```python
from build123d import *

# Parameters (mm, degrees)
BOSS_EXTRUDE1_DEPTH = 50.8
SKETCH3_R           = 3.302
CUT_EXTRUDE1_DEPTH  = 50.8
SKETCH4_R           = 3.302
CUT_EXTRUDE2_DEPTH  = 70.633186233


with BuildPart() as part:
    # Sketch2 → Boss-Extrude1 (new body)
    with BuildSketch(Plane(origin=(0, 0, 0), x_dir=(1, 0, 0), z_dir=(0, 1, 0))):
        Polygon((0, 0), (0, -28.575), (38.1, -28.575), (38.1, 0), (34.925, 0), (34.925, -25.4), (3.175, -25.4), (3.175, 0), align=None)
    extrude(amount=BOSS_EXTRUDE1_DEPTH)

    # Sketch3 → Cut-Extrude1 (cut)
    with BuildSketch(Plane(origin=(0, 0, 25.4), x_dir=(-1, 0, 0), z_dir=(0, 0, -1))):
        with Locations((-19.685, 12.7)):
            Circle(SKETCH3_R)
        with Locations((-19.685, 38.091107032)):
            Circle(SKETCH3_R)
    extrude(amount=-CUT_EXTRUDE1_DEPTH, mode=Mode.SUBTRACT)

    # Sketch4 → Cut-Extrude2 (cut, through all)
    with BuildSketch(Plane(origin=(38.1, 0, 0), x_dir=(0, 0, -1), z_dir=(1, 0, 0))):
        with Locations((-11.90625, 38.1)):
            Circle(SKETCH4_R)
        with Locations((-11.90625, 12.7)):
            Circle(SKETCH4_R)
    extrude(amount=-CUT_EXTRUDE2_DEPTH, mode=Mode.SUBTRACT)


solid = part.part
```
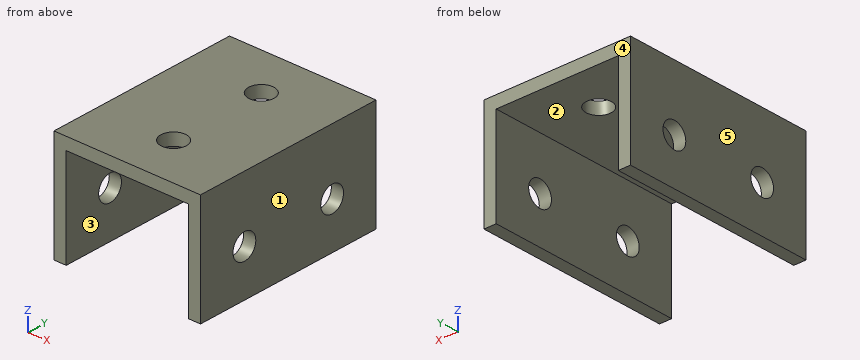
Can you work these out from the model? Positions are in its coordinate system, mm. Face numbers are marked on the shaded views. A direction names the side the tool comes from. Coordinates: 2 decimals unless noted, no trailing zeros. Order: outer loops, then holes, each group sorted by start corner. A loop starts at its lowest first (then second) coordinate and runs counter-clockwise, first axis right, second up. Notation, with made-up numbers: (36, -14.5) -> (42, -14.5) arc R22 ccw to (42, 1.5) -> close; hole circle Ø2 at (-33, 82). An arc over 180 degrees is marked (long way). Write each question's results on one line, items separated by ' | '.
Item 1: I want a section at B-B, the plane y = 12.7. Write out the boundary of the cut face in (x, z) (3 decimals), then the cut area to 3 significant figures.
Results are:
outline: (0, 0) -> (3.175, 0) -> (3.175, 8.604) -> (0, 8.604) -> close; (0, 15.208) -> (3.175, 15.208) -> (3.175, 25.4) -> (16.383, 25.4) -> (16.383, 28.575) -> (0, 28.575) -> close; (22.987, 25.4) -> (34.925, 25.4) -> (34.925, 15.208) -> (38.1, 15.208) -> (38.1, 28.575) -> (22.987, 28.575) -> close; (34.925, 0) -> (38.1, 0) -> (38.1, 8.604) -> (34.925, 8.604) -> close | area: 219 mm²
Item 2: If I drill on line 1 along X through (y, z) = (31, 21.5) (3 decimals); line 2 along Z through (x, y) = (24.5, 49) (3 decimals), over which ranges is the centre line in solid material (lowest first)?
Results are:
line 1: 0 to 3.175, 34.925 to 38.1 | line 2: 25.4 to 28.575
Item 3: I want a section at D-D, the plane y = 24. Write out the boundary of the cut face in (x, z) (3 decimals).
Results are:
outline: (0, 0) -> (3.175, 0) -> (3.175, 25.4) -> (34.925, 25.4) -> (34.925, 0) -> (38.1, 0) -> (38.1, 28.575) -> (0, 28.575) -> close
Item 4: I'm going to push flat-ended pins straight in: pin 1 Ø8.5 at (x, y) = (19.685, 12.7) entering from +Z (3 decimals); pin 2 Ø4 at (y, z) = (12.7, 11.91) entering from +X; pin 3 Ø12 at (x, y) = (25.5, 19) entering from -Z. Where does each tip first touch, or does it pass through?
Results are:
pin 1: z = 28.575 | pin 2: through | pin 3: z = 25.4
Item 5: I want a section at C-C, the plane x = 22. Write out the boundary of the cut face in (y, z) (3 decimals).
Results are:
outline: (0, 25.4) -> (10.345, 25.4) -> (10.345, 28.575) -> (0, 28.575) -> close; (15.055, 25.4) -> (35.737, 25.4) -> (35.737, 28.575) -> (15.055, 28.575) -> close; (40.446, 25.4) -> (50.8, 25.4) -> (50.8, 28.575) -> (40.446, 28.575) -> close
Item 6: Which directions (+Z, -Z, +X, -X, +Y, -Y) give clear straight access to the entire face, cutting with the end or side of a thin tool? Please do the marked faces 1 and 2.
Results are:
face 1: +Z, -Z, +X, +Y, -Y | face 2: -Z, +Y, -Y
Item 7: I want a section at A-A, the plane z = 6. Write out the boundary of the cut face in (x, y) (3 decimals), then the cut area to 3 significant figures.
Results are:
outline: (0, 0) -> (3.175, 0) -> (3.175, 50.8) -> (0, 50.8) -> close; (34.925, 0) -> (38.1, 0) -> (38.1, 50.8) -> (34.925, 50.8) -> close | area: 323 mm²
Item 8: If we mould it in two halves opening along X, with no side actions, what happens to the marked faces 3, 4 and 5? For each: +X half, -X half, draft (parallel to the pull), parting line (faces both ways), or undercut.
Results are:
face 3: undercut | face 4: draft | face 5: -X half
